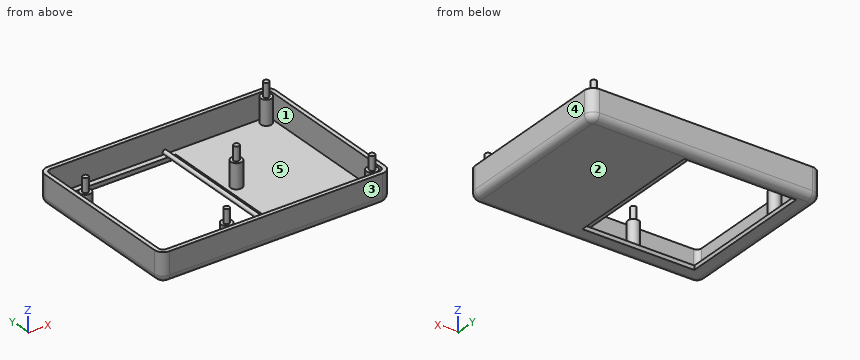
```python
from build123d import *

# Parameters (mm, degrees)
F1_DEPTH  = 21
F2_T      = -3
F3_R      = 5.08
F4_R      = 4
F5_DEPTH  = 17.5
F6_R      = 1.95
F7_DEPTH  = 10
F8_W      = 80
F8_H      = 100
F9_DEPTH  = 25
F10_R     = 1.5
F11_DEPTH = 115


with BuildPart() as f1:
    # F0 (on Top) → F1 (new body)
    with BuildSketch(Plane.XY):
        with BuildLine():
            ThreePointArc((-83.334517, -38.901611), (-81.474645, -43.391739), (-76.984517, -45.251611))
            Line((-76.984517, -45.251611), (75.315483, -45.251611))
            ThreePointArc((75.315483, -45.251611), (79.805611, -43.391739), (81.665483, -38.901611))
            Line((81.665483, -38.901611), (81.665483, 68.398389))
            ThreePointArc((81.665483, 68.398389), (79.805611, 72.888517), (75.315483, 74.748389))
            Line((75.315483, 74.748389), (-76.984517, 74.748389))
            ThreePointArc((-76.984517, 74.748389), (-81.474645, 72.888517), (-83.334517, 68.398389))
            Line((-83.334517, 68.398389), (-83.334517, -38.901611))
        make_face()
    extrude(amount=F1_DEPTH)

    # F2
    f2_openings = [f1.faces().sort_by_distance(p)[0] for p in [
        (-0.834517, 14.748389, 21),
    ]]
    offset(amount=F2_T, openings=f2_openings)

    # F3
    f3_edges = [f1.edges().sort_by_distance(p)[0] for p in [
        (-81.474645, 72.888517, 0),
    ]]
    fillet(f3_edges, radius=F3_R)

    # F4 (on face) → F5 (join)
    with BuildSketch(Plane.XY.offset(3)):
        with Locations((73.665483, -37.251611)):
            Circle(F4_R)
        with Locations((73.665483, 66.748389)):
            Circle(F4_R)
        with Locations((16.665483, 17.748389)):
            Circle(F4_R)
        with Locations((-75.334517, 39.748389)):
            Circle(F4_R)
        with Locations((-30.334517, -37.251611)):
            Circle(F4_R)
    extrude(amount=F5_DEPTH)

    # F6 (on face) → F7 (join)
    with BuildSketch(Plane.XY.offset(20.5)):
        with Locations((73.665483, -37.251611)):
            Circle(F6_R)
        with Locations((16.665483, 17.748389)):
            Circle(F6_R)
        with Locations((73.665483, 66.748389)):
            Circle(F6_R)
        with Locations((-30.334517, -37.251611)):
            Circle(F6_R)
        with Locations((-75.334517, 39.748389)):
            Circle(F6_R)
    extrude(amount=F7_DEPTH)

    # F8 (on face) → F9 (cut)
    with BuildSketch(Plane(origin=(0, 0, 0), x_dir=(1, 0, 0), z_dir=(0, 0, -1))):
        with Locations((-30.334517, -17.748389)):
            Rectangle(F8_W, F8_H)
    extrude(amount=-F9_DEPTH, mode=Mode.SUBTRACT)

    # F10 (on face) → F11 (join)
    with BuildSketch(Plane.XZ.offset(-71.748389)):
        with Locations((4.665483, 4.55)):
            Circle(F10_R)
    extrude(amount=F11_DEPTH)


solid = f1.part
```
Input: part model. Units: mm. Frame: model coordinates. Face numbers are marked on the shaded views. A direction names the side the tool comes from. Round coordinates to 2 decimals unless told otherwise and drop trailing zeros. Write each loop counter-clockwise with the first axis right and the second up, starting at its lowest first coordinate (ties: lowest second). Pieces come first, ordered by that corner, then holes. Notation, with made-up numbers: (6, 35.25) -> (51, 35.25) arc R14 cw to (51, 46.25) -> close; hole circle Ø11 at (-36, 24.5). An arc over 180 degrees is marked (long way). Answer as CSV lines item,"result".
1. Section D-D (x = 47). Return the cut outline in (y, z).
Geometry says:
outline,"(-45.25, 5.08) arc R5.08 ccw to (-40.17, 0) -> (69.67, 0) arc R5.08 ccw to (74.75, 5.08) -> (74.75, 21) -> (71.75, 21) -> (71.75, 3) -> (-42.25, 3) -> (-42.25, 21) -> (-45.25, 21) -> close"
2. Contact query for flat-ended pins moving along their axis: P1, Ø3.5, axis at x = -27, z = 1.5, coming from the +Y side; P2, Ø3.5, axis at y = 24, z = 1.5, coming from the +X side; P3, Ø0.9, axis at x = -36.5, z = 1.5, coming from the -Y side. Output: stop coordinate, or through.
Geometry says:
P1,"stops at y = 74.41"
P2,"stops at x = 81.32"
P3,"stops at y = -44.17"
3. Mould query, pull axis Y, two halves, no side actions, for the marked faces 3, 4 and 5. Classes: +Y half, -Y half, draft (parallel to the pull), parting line (faces both ways), or undercut.
Geometry says:
face 3,"-Y half"
face 4,"draft"
face 5,"undercut"
4. Section A-A (x = -41.5). Return the cut outline in (y, z).
Geometry says:
outline,"(-45.25, 5.08) arc R5.08 ccw to (-40.17, 0) -> (-32.25, 0) -> (-32.25, 3) -> (-42.25, 3) -> (-42.25, 21) -> (-45.25, 21) -> close; (67.75, 0) -> (69.67, 0) arc R5.08 ccw to (74.75, 5.08) -> (74.75, 21) -> (71.75, 21) -> (71.75, 3) -> (67.75, 3) -> close"
5. Section C-C (z = 9). Return the cut outline in (x, y), plus the area to 3 significant figures.
Geometry says:
outline,"(-83.33, -38.9) arc R6.35 ccw to (-76.98, -45.25) -> (75.32, -45.25) arc R6.35 ccw to (81.67, -38.9) -> (81.67, 68.4) arc R6.35 ccw to (75.32, 74.75) -> (-76.98, 74.75) arc R6.35 ccw to (-83.33, 68.4) -> close; circle Ø8 at (-75.33, 39.75); circle Ø8 at (-30.33, -37.25); circle Ø8 at (16.67, 17.75); circle Ø8 at (73.67, -37.25); circle Ø8 at (73.67, 66.75); hole (-80.33, -38.9) arc R3.35 ccw to (-76.98, -42.25) -> (75.32, -42.25) arc R3.35 ccw to (78.67, -38.9) -> (78.67, 68.4) arc R3.35 ccw to (75.32, 71.75) -> (-76.98, 71.75) arc R3.35 ccw to (-80.33, 68.4) -> close"
area,"1,900 mm^2"
6. Section B-B (y = -8). Return the cut outline in (x, z).
Geometry says:
outline,"(-83.33, 5.08) arc R5.08 ccw to (-78.25, 0) -> (-70.33, 0) -> (-70.33, 3) -> (-80.33, 3) -> (-80.33, 21) -> (-83.33, 21) -> close; circle Ø3 at (4.67, 4.55); (9.67, 0) -> (76.59, 0) arc R5.08 ccw to (81.67, 5.08) -> (81.67, 21) -> (78.67, 21) -> (78.67, 3) -> (9.67, 3) -> close"
7. Reachability of the marked faces 1 and 2 from +Z, -Z, +X, -X, +Y, -Y: full face, straight path, thin tool, end or side. Return the list, or none.
Geometry says:
face 1,"+Z"
face 2,"-Z, +X, -X, +Y, -Y"
8. Ray query, L1, parallel to X at y = -19, z = 10; L2, parallel to Y at x = -25.5, z = 13.5; L3, parallel to X at y = 66, z = 15. Return the intervals inside material, ascending. Write a range as [from, to].
Geometry says:
L1,"x = [-83.33, -80.33], [78.67, 81.67]"
L2,"y = [-45.25, -42.25], [71.75, 74.75]"
L3,"x = [-83.33, -80.33], [69.74, 77.59], [78.67, 81.67]"
